Study the drawing (mm; zero at the part's minimum x, y, z) and answer. Coordinates: 2 decimals unless noted, no trailing zeros. Write each loop counter-clockwise with the first axis right and the second up, starting at its lowest first coordinate (ties: lowest second). Pieces come first, ordered by that corner, then holes. Notation, with made-up numbers: M 43.25,72.5 L 86.25,72.5 A36 cw 86.25,108.5 Z; hole C 79.25,51.5 d6. An arc over 180 degrees is marked long. Answer as CSV lines item,"result". Start each with the question number.
(1) A cutting plane is placed at B-B on z = 2.5. Give the vertices of the cut face in (x, y).
(2) Find the intervals of material crossed by L1, parallel to Y at x = 116, z = 1.1; L2, parallel to X at y = 51, z = 1.1 (1 decimal); L3, parallel to X at y = 42.5, z = 2.4, in increasing order. Write a range as [from, to].
(3) A cutting plane is placed at C-C on y = 32.5. Give the vertices of the cut face in (x, z), then the cut area to 3 significant figures.
(4) Flat-ended cylindrical pins translate along their axes: P1, Ø2.5, axis at x = 55.87, y = 66.32, coming from the -Z side; P2, Ø1.2, axis at x = 106.67, y = 51.02, coming from the -Z side; P3, Ø2, axis at x = 131.5, z = 2, coming from the +Y side; P4, Ø1.2, axis at x = 128, z = 2.5, coming from the -Y side. Find the tip coordinate at first contact, or state that the pin passes through.
(5) The mould has two halves that part along Z. Classify the marked faces 1 and 2: released by +Z, released by -Z, zero draft, split by the parting line, or undercut.
(6) A cutting plane is placed at A-A on x = 138. Give the vertices of the cut face in (y, z).
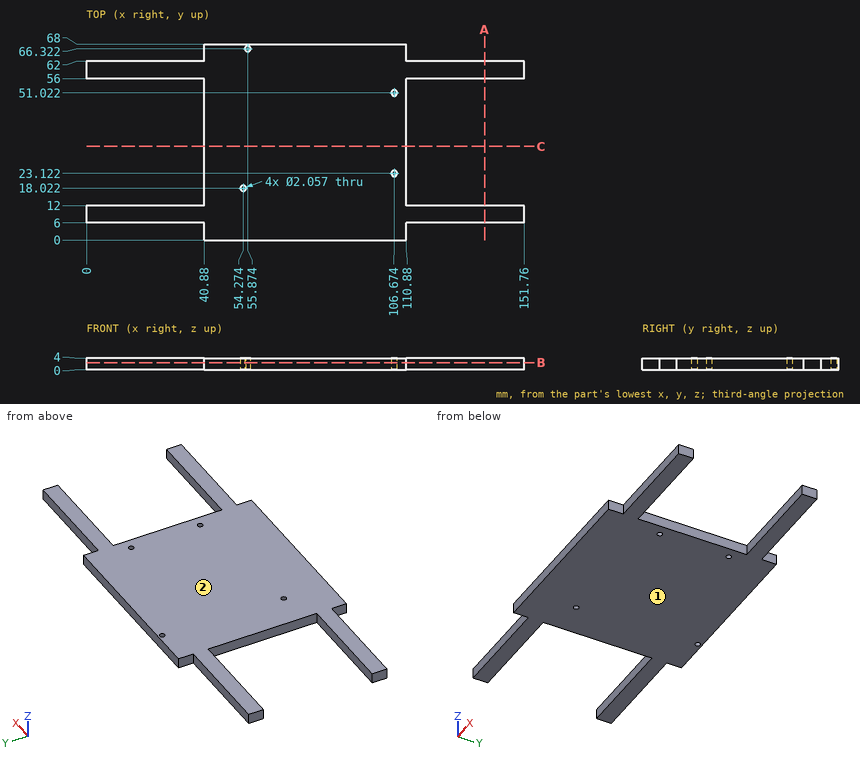
Here are the results:
1,outline,"M 0,6 L 40.88,6 L 40.88,0 L 110.88,0 L 110.88,6 L 151.76,6 L 151.76,12 L 110.88,12 L 110.88,56 L 151.76,56 L 151.76,62 L 110.88,62 L 110.88,68 L 40.88,68 L 40.88,62 L 0,62 L 0,56 L 40.88,56 L 40.88,12 L 0,12 Z; hole C 54.27,18.02 d2.06; hole C 55.87,66.32 d2.06; hole C 106.67,23.12 d2.06; hole C 106.67,51.02 d2.06"
2,L1,"y = [6, 12], [56, 62]"
2,L2,"x = [40.9, 105.6], [107.7, 110.9]"
2,L3,"x = [40.88, 110.88]"
3,outline,"M 40.88,0 L 110.88,0 L 110.88,4 L 40.88,4 Z"
3,area,"280 mm^2"
4,P1,"stops at z = 0"
4,P2,"passes through"
4,P3,"stops at y = 62"
4,P4,"stops at y = 6"
5,face 1,"released by -Z"
5,face 2,"released by +Z"
6,outline,"M 6,0 L 12,0 L 12,4 L 6,4 Z; M 56,0 L 62,0 L 62,4 L 56,4 Z"
